Could you check a few things on this model? Use its own coordinates, in mm. A direction names the side the tool comes from. Give positions to 0.01 mm unless a question says otherwise; leave off trailing zeros. Order: outer loops, then holes, each group sorted by start corner. A loop starts at its lowest first (then second) coordinate and runs counter-clockwise, first axis right, second up.
(1) If we mould it in two halves opening along X, with no side actions, what happens to faces 6 (the flat face through (37, 11, 2)), 7 (the flat face through (71, -25, 2)), 8 (the cylindrical face through (-69.9, 22.8, 3.5)), 9 (the flat face through (66, 0.05, 2))? For each: released by +X, released by -X, zero draft, split by the parting line, or undercut.
(2) Will these pins go through, and if not, where does the flat tip stop? pin 1 (3 mm diameter, centred on x = -15, z = 2.5, fed in from +Y); pin 2 (7.5 mm diameter, centred on x = 45, y = -1, fed in from +Z); pin 3 (1.2 mm diameter, centred on x = 22, z = 3, fed in from +Y).
(3) Imagine slicing it at A-A, the plane x = -67.5. Write out the boundary of the cut face in (y, z), then the cut area to 3 significant figures.
(4) If I drill on probe 1 along Y at (x, z) = (-67.5, 3.85); probe 2 along X at (y, z) = (16.5, 4.2); probe 3 along Y at (x, z) = (-67.5, 1), over which ranges is the centre line in solid material (lowest first)?
(5) On a 3-axis mill with a long thin cutter (end or side, diameter ignored), from which of +Z, -Z, +X, -X, +Y, -Y can I reach the whole of each face in a straight line? I mean faces 1 (the flat face through (-45.05, -24, 2)), 2 (the flat face through (67.55, -7, 2)), 3 (the flat face through (-59, 26, 2)), 4 (the flat face through (-46, -4, 1)), 5 (the flat face through (2.5, 19, 2)). Say none if no direction works.
(6) Imagine slicing it at D-D, the plane y = 13. Write out the boundary of the cut face in (x, z).
(7) Imagine slicing it at C-C, the plane x = 29. Write out the boundary of the cut face in (y, z).
(8) Imagine slicing it at B-B, the plane y = -5. Write out the boundary of the cut face in (x, z), then the cut area to 3 significant figures.
Autodesk Inventor part; units mm, degrees
ref_plane "YZ Plane" through (0, 0, 0) normal (1, 0, 0) x (0, 1, 0)
ref_plane "XZ Plane" through (0, 0, 0) normal (0, 1, 0) x (-1, 0, 0)
ref_plane "XY Plane" through (0, 0, 0) normal (0, 0, 1) x (1, 0, 0)
sketch "スケッチ2" plane through (-42.95, -23, 0) normal (0, -1, 0) x (1, 0, 0)
  line L0 (0, 0) -> (25.9, 5) construction
  line L1 (0, 5) -> (25.9, 5)
  line L2 (12.95, 5) -> (12.95, 0) construction
  line L3 (0, 0) -> (25.9, 0)
  line L4 (0, 0) -> (0, 5)
  line L5 (0, 2.5) -> (25.9, 2.5) construction
  line L6 (25.9, 0) -> (25.9, 5)
  point P0 (42.95, 0)
  point P1 (2.95, 2.5)
  point P2 (22.95, 2.5)
  dimension "d176" = 20
sketch "スケッチ1" plane through (0, 0, 0) normal (0, 0, 1) x (1, 0, 0)
  line L0 (-72.5, 26) -> (-47.1, 26)
  line L1 (72.5, 26) -> (72.5, 11) construction
  line L2 (-72.5, -26) -> (-72.5, 26)
  line L3 (-72.5, 26) -> (72.5, -26) construction
  line L4 (72.5, 26) -> (-72.5, -26) construction
  line L5 (2.5, 26) -> (2.5, 11)
  line L6 (2.5, 11) -> (4.6, 11) construction
  line L7 (2.5, 26) -> (72.5, 26) construction
  line L8 (72.5, 11) -> (72.5, -26)
  line L9 (70, 11) -> (70, -26) construction
  circle A0 centre (67.5, 6) radius 1.55
  line L10 (-45, 26) -> (-45, 31)
  line L11 (-45, 31) -> (-25, 31)
  line L12 (-25, 31) -> (-25, 26)
  line L13 (-45, 26) -> (-25, 26) construction
  line L14 (-25, 26) -> (-22.9, 26) construction
  arc A1 (-47.1, 26) -> (-45, 26) centre (-46.05, 26) ccw
  arc A2 (-25, 26) -> (-22.9, 26) centre (-23.95, 26) ccw
  line L15 (-47.1, 26) -> (-45, 26) construction
  line L16 (-22.9, 26) -> (2.5, 26)
  line L17 (65, 11) -> (65, -26) construction
  line L18 (-45.05, -23) -> (-45.05, -26)
  line L19 (-14.95, -23) -> (-14.95, -26)
  line L20 (-45.05, -23) -> (-42.95, -23) construction
  arc A3 (-42.95, -23) -> (-45.05, -23) centre (-44, -23) ccw
  arc A4 (-14.95, -23) -> (-17.05, -23) centre (-16, -23) ccw
  line L21 (-42.95, -23) -> (-17.05, -23)
  line L22 (-17.05, -23) -> (-14.95, -23) construction
  line L23 (15, -23) -> (45, -23) construction
  line L24 (45, -23) -> (45, -24.5) construction
  line L25 (45, -24.5) -> (15, -24.5) construction
  line L26 (15, -24.5) -> (15, -23) construction
  line L27 (15, -23) -> (45, -24.5) construction
  line L28 (45, -23) -> (15, -24.5) construction
  line L29 (14.95, -22.95) -> (45.05, -22.95)
  line L30 (45.05, -22.95) -> (45.05, -24.55) construction
  line L31 (45.05, -24.55) -> (14.95, -24.55)
  line L32 (14.95, -24.55) -> (14.95, -22.95) construction
  line L33 (14.95, -22.95) -> (45.05, -24.55) construction
  line L34 (45.05, -22.95) -> (14.95, -24.55) construction
  line L35 (-45, -23) -> (-45, -26) construction
  line L36 (-15, -23) -> (-15, -26) construction
  line L37 (72.5, -7.5) -> (-72.5, -7.5) construction
  line L38 (67.5, 0) -> (65, 0) construction
  line L39 (65, 0) -> (65, -15) construction
  line L40 (65, -15) -> (67.5, -15) construction
  line L41 (67.5, -15) -> (67.5, 0) construction
  line L42 (67.5, 0) -> (65, -15) construction
  line L43 (65, 0) -> (67.5, -15) construction
  line L44 (64.95, 0.05) -> (67.55, 0.05)
  line L45 (67.55, 0.05) -> (67.55, -2.05) construction
  line L46 (67.55, -15.05) -> (64.95, -15.05)
  line L47 (64.95, -15.05) -> (64.95, -12.95) construction
  line L48 (64.95, 0.05) -> (67.55, -15.05) construction
  line L49 (67.55, 0.05) -> (64.95, -15.05) construction
  arc A5 (64.95, 0.05) -> (64.95, -2.05) centre (64.95, -1) ccw
  arc A6 (67.55, -2.05) -> (67.55, 0.05) centre (67.55, -1) ccw
  arc A7 (64.95, -12.95) -> (64.95, -15.05) centre (64.95, -14) ccw
  arc A8 (67.55, -15.05) -> (67.55, -12.95) centre (67.55, -14) ccw
  line L50 (64.95, -2.05) -> (64.95, 0.05) construction
  line L51 (64.95, -12.95) -> (64.95, -2.05)
  line L52 (67.55, -12.95) -> (67.55, -15.05) construction
  line L53 (67.55, -2.05) -> (67.55, -12.95)
  arc A9 (14.95, -22.95) -> (14.95, -24.55) centre (14.95, -23.75) ccw
  arc A10 (45.05, -24.55) -> (45.05, -22.95) centre (45.05, -23.75) ccw
  circle A11 centre (67.5, -21) radius 1.55
  line L54 (-72.5, -26) -> (-45, -26)
  line L55 (-15, -26) -> (72.5, -26)
  line L56 (-45, -26) -> (-15, -26) construction
  line L57 (-70, 26) -> (-70, -26) construction
  line L58 (-65, 26) -> (-65, -26) construction
  arc A12 (2.5, 11) -> (4.6, 11) centre (3.55, 11) ccw
  line L59 (4.6, 11) -> (72.5, 11)
  circle A13 centre (67.5, 6) radius 3
  circle A14 centre (67.5, -21) radius 3
  line L60 (2.5, 6) -> (2.5, -18)
  line L61 (2.5, -18) -> (46.579, -18)
  line L62 (46.579, -18) -> (6.0385, 6)
  line L63 (15.8534, 6) -> (60, 6)
  line L64 (60, 6) -> (60, -20.1348)
  line L65 (60, -20.1348) -> (15.8534, 6)
  line L66 (-65, 17.7579) -> (-65, -18)
  line L67 (-65, -18) -> (-13.4261, -18)
  line L68 (-13.4261, -18) -> (-65, 17.7579)
  line L69 (-60.9008, 21) -> (-2.5, 21)
  line L70 (-2.5, 21) -> (-2.5, -19.4912)
  line L71 (-2.5, -19.4912) -> (-60.9008, 21)
  line L72 (-72.5, 26) -> (2.5, -26) construction
  line L73 (2.5, 11) -> (2.5, -26) construction
  line L74 (6.0385, 6) -> (2.5, 6)
  line L75 (2.5, 11) -> (65, -26) construction
  circle A15 centre (-67.5, 21) radius 1.25
  circle A16 centre (-67.5, 21) radius 3
  circle A17 centre (-67.5, -23.5) radius 1.5
  circle A18 centre (-67.5, -18.5) radius 1.5
  circle A19 centre (-67.5, -13.5) radius 1.5
  line L76 (-67.5, 26) -> (-67.5, -26) construction
  point P0 (0, 0)
  point P1 (30, -23.75)
  point P2 (66.25, -7.5)
  dimension "d0" = 145
  dimension "d1" = 52
  dimension "d2" = 75
  dimension "d3" = 15
  dimension "d4" = 2.5
  dimension "d5" = 3.1
  dimension "d6" = 2.5
  dimension "d7" = 5
  dimension "d12" = 20
  dimension "d13" = 27.5
  dimension "d14" = 5
  dimension "d15" = 1.05
  dimension "d16" = 1.05
  dimension "d17" = 70
  dimension "d55" = 1.05
  dimension "d56" = 1.05
  dimension "d74" = 37
  dimension "d107" = 30
  dimension "d108" = 1.5
  dimension "d109" = 0.05
  dimension "d110" = 0.05
  dimension "d114" = 0.05
  dimension "d115" = 0.05
  dimension "d116" = 30
  dimension "d118" = 5
  dimension "d123" = 2.5
  dimension "d124" = 15
  dimension "d125" = 0.05
  dimension "d126" = 0.05
  dimension "d127" = 1.05
  dimension "d128" = 1.05
  dimension "d129" = 1.05
  dimension "d130" = 1.05
  dimension "d132" = 30
  dimension "d133" = 20
  dimension "d134" = 3
  dimension "d135" = 2.5
  dimension "d146" = 5
  dimension "d147" = 20
  dimension "d148" = 130
  dimension "d152" = 1.05
  dimension "d169" = 6
  dimension "d185" = 5
  dimension "d186" = 5
  dimension "d187" = 5
  dimension "d188" = 2.5
  dimension "d190" = 8
  dimension "d191" = 5
  dimension "d192" = 5
  dimension "d193" = 5
  dimension "d195" = 5
  dimension "d196" = 2.5
  dimension "d200" = 2.5
  dimension "d201" = 6
  dimension "d204" = 5
  dimension "d205" = 2.5
  dimension "d206" = 3
  dimension "d207" = 3
  dimension "d208" = 3
  dimension "d209" = 2.5
  dimension "d210" = 2.5
  dimension "d211" = 5
  dimension "d212" = 5
extrude "押し出し1" add sketch "スケッチ1" along normal blind 5 contours L0 A1 L10 L11 L12 A2 L16 L5 A12 L59 L8 L55 L19 A4 L21 A3 L18 L54 L2
extrude "押し出し2" add sketch "スケッチ1" along normal blind 2 contours A13 | A14 | A16
hole "穴1" at (-40, -23, 2.5) at (-20, -23, 2.5) direction (0, 1, 0) diameter 2.459 depth 5
chamfer "面取り1" distance 2.5 angle 45 4 edges at (72.5, -26, 2.5) (72.5, 11, 2.5) (-72.5, 26, 2.5) (-72.5, -26, 2.5)
sketch "スケッチ3" plane through (-47.1, 26, 5) normal (0, 1, 0) x (1, 0, 0)
  line L0 (22.1, 0) -> (2.1, 0)
  line L1 (12.1, 0) -> (12.1, 5) construction
  line L2 (22.1, 5) -> (2.1, 5)
  line L3 (-22.9, 0) -> (-22.9, 5)
  line L4 (-22.9, 2.5) -> (49.6, 2.5) construction
  line L5 (49.6, 5) -> (49.6, 0)
  point P0 (47.1, 5)
  point P1 (-7.9, 2.5)
  point P2 (32.1, 2.5)
  dimension "d177" = 40
hole "穴2" at (-55, 26, 2.5) at (-15, 26, 2.5) direction (0, -1, 0) diameter 2.459 depth 5
fillet "フィレット2" radius 1 13 edges at (-65, 17.7579, 2.5) (-60.9008, 21, 2.5) (-2.5, 21, 2.5) (-65, -18, 2.5) (-13.4261, -18, 2.5) (-2.5, -19.4912, 2.5) (2.5, -18, 2.5) (2.5, 6, 2.5) (6.0385, 6, 2.5) (15.8534, 6, 2.5) (60, 6, 2.5) (60, -20.1348, 2.5) (46.579, -18, 2.5)
extrude "押し出し4" add sketch "スケッチ1" along normal blind 1 contours L74 L62 L61 L60 | L63 L64 L65 | L68 L67 L66 | L69 L70 L71
equation "\"d13\" = -0.5 * d12 + 0.5 * d2"
equation "\"d16\" = d15"
equation "\"d55\" = d54"
equation "\"d56\" = d55"
equation "\"d53\" = d15"
equation "\"d54\" = d53"
properties part number "Cockpit_vertical_frame_03" material "アセタール樹脂、黒"
Answer block:
1. face 6: zero draft
1. face 7: released by +X
1. face 8: undercut
1. face 9: undercut
2. pin 1: stops at y = 26
2. pin 2: stops at z = 1
2. pin 3: stops at y = 11
3. outline: (-26, 0) - (-25, 0) - (-25, 5) - (-26, 5) - close; (-22, 0) - (-20, 0) - (-20, 5) - (-22, 5) - close; (-17, 0) - (-15, 0) - (-15, 5) - (-17, 5) - close; (-12, 0) - (19.75, 0) - (19.75, 2) - (18, 2) - (18, 5) - (-12, 5) - close; (22.25, 0) - (26, 0) - (26, 5) - (24, 5) - (24, 2) - (22.25, 2) - close
3. area: 192 mm2
4. probe 1: y = -26 to -25, -22 to -20, -17 to -15, -12 to 18, 24 to 26
4. probe 2: x = -72.5 to -64.76, -63.19 to -54.41, -2.5 to 2.5
4. probe 3: y = -26 to -25, -22 to -20, -17 to -15, -12 to 19.75, 22.25 to 26
5. face 1: +Z, -Z, -Y
5. face 2: +Z, -Z
5. face 3: +Z, -Z, -X, +Y
5. face 4: +Z
5. face 5: +Z, -Z, +X, +Y
6. outline: (-72.5, 0) - (2.5, 0) - (2.5, 5) - (-2.5, 5) - (-2.5, 1) - (-49.36, 1) - (-49.36, 5) - (-58.14, 5) - (-58.14, 1) - (-65, 1) - (-65, 5) - (-72.5, 5) - close
7. outline: (-26, 0) - (-24.55, 0) - (-24.55, 5) - (-26, 5) - close; (-22.95, 0) - (11, 0) - (11, 5) - (6, 5) - (6, 1) - (-1.78, 1) - (-1.78, 5) - (-7.59, 5) - (-7.59, 1) - (-18, 1) - (-18, 5) - (-22.95, 5) - close
8. outline: (-72.5, 0) - (64.95, 0) - (64.95, 5) - (60, 5) - (60, 1) - (34.43, 1) - (34.43, 5) - (24.62, 5) - (24.62, 1) - (2.5, 1) - (2.5, 5) - (-2.5, 5) - (-2.5, 1) - (-23.4, 1) - (-23.4, 5) - (-32.18, 5) - (-32.18, 1) - (-65, 1) - (-65, 5) - (-72.5, 5) - close; (67.55, 0) - (72.5, 0) - (72.5, 5) - (67.55, 5) - close
8. area: 306 mm2
